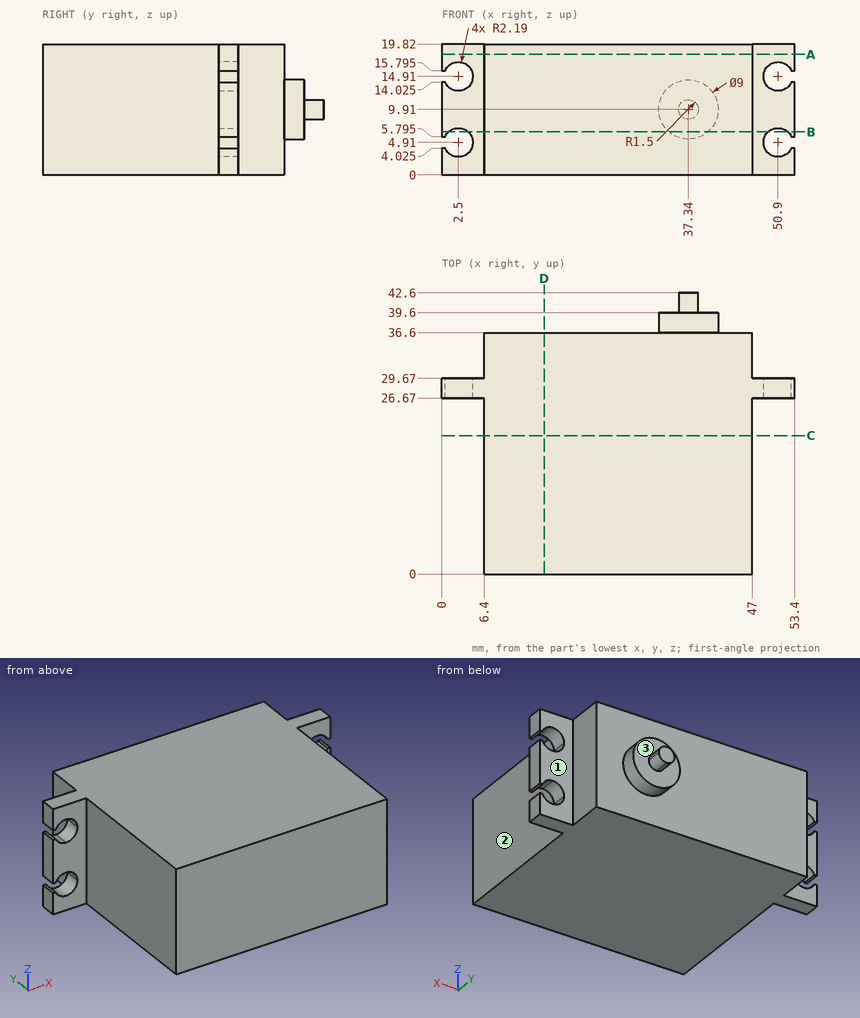
Geometry: see drawing. Coordinates: mm, zero at the bounding-box minimum. A direction names the side the tool comes from. Round coordinates to 2 decimals unless told otherwise and drop trailing zeros. Order: outer loops, then holes, each group sorted by start corner. A loop starts at its lowest first (then second) coordinate and runs counter-clockwise, first axis right, second up. Notation, with made-up numbers: (51.5, 19.25) -> (73.5, 19.25) arc R13 ccw to (73.5, 38.25) -> close; hole circle Ø2 at (46.5, -13.5). An arc over 180 degrees is marked (long way). Write each question's results on one line, items separated by ' | '.
Q1. Section query D-D (x = 15.5). Output: boundary loops of the cut face in (y, z), and give its area (3 significant figures).
Response values:
outline: (0, 0) -> (36.6, 0) -> (36.6, 19.82) -> (0, 19.82) -> close | area: 725 mm²
Q2. Access query for the marked faces 1, 2 and 3. Directions: +Z, -Z, +X, -X, +Y, -Y. A direction counts if a zero-diameter tool reaches every point of the face in a straight line with its end or side. Return the directions, or none.
Response values:
face 1: +Z, -Z, +X, +Y | face 2: +Z, -Z, +X, -Y | face 3: +Y
Q3. Ray query, line 1 along X through (y, z) = (13.5, 18.5); line 2 along Y through (x, z) = (19.5, 18); line 3 along Y through (x, z) = (49, 3.75). Return the intervals inside material, ascending.
Response values:
line 1: 6.4 to 47 | line 2: 0 to 36.6 | line 3: 26.67 to 29.67
Q4. Section query C-C (y = 21). Output: boundary loops of the cut face in (x, z), and give its area (3 significant figures).
Response values:
outline: (6.4, 0) -> (47, 0) -> (47, 19.82) -> (6.4, 19.82) -> close | area: 805 mm²
Q5. Pin query (flat end, axial travel): pin 1 Ø3 at (x, z) = (49, 12.5) entering from +Y; pin 2 Ø5 at (x, z) = (50, 8) entering from -Y; pin 3 Ø1.5 at (y, z) = (13, 11.5) entering from -X. Return the tip coordinate at first contact, or that it passes through.
Response values:
pin 1: y = 29.67 | pin 2: y = 26.67 | pin 3: x = 6.4
Q6. Section query B-B (z = 6.5). Output: boundary loops of the cut face in (x, y).
Response values:
outline: (0, 26.67) -> (0.99, 26.67) -> (0.99, 29.67) -> (0, 29.67) -> close; (4.01, 26.67) -> (6.4, 26.67) -> (6.4, 0) -> (47, 0) -> (47, 26.67) -> (49.39, 26.67) -> (49.39, 29.67) -> (47, 29.67) -> (47, 36.6) -> (40.28, 36.6) -> (40.28, 39.6) -> (34.4, 39.6) -> (34.4, 36.6) -> (6.4, 36.6) -> (6.4, 29.67) -> (4.01, 29.67) -> close; (52.41, 26.67) -> (53.4, 26.67) -> (53.4, 29.67) -> (52.41, 29.67) -> close
Q7. Section query A-A (z = 18.25). Output: boundary loops of the cut face in (x, y), and give its area (3 significant figures).
Response values:
outline: (0, 26.67) -> (6.4, 26.67) -> (6.4, 0) -> (47, 0) -> (47, 26.67) -> (53.4, 26.67) -> (53.4, 29.67) -> (47, 29.67) -> (47, 36.6) -> (6.4, 36.6) -> (6.4, 29.67) -> (0, 29.67) -> close | area: 1,520 mm²
